For this review, take the finished solid that the model builds, in its own axes (mm). Give positions to 0.01 mm unless a question says otherwise; leave off trailing zeros. Loops run counter-clockwise (first coordinate to the right, second up) from the corner with the lowest first, then second, coordinate; pieces in that order, holes last. Notation, with made-up numbers: M -38,76.5 L 14,76.5 A6 ccw 14,86.5 Z; hole C -4.5,61.25 d3. An arc over 180 degrees is marked long. Use CSV: the item, a comma, the result in double quotes. Start each with the question number.
1. Take a section at C-C, the plane x = -6. Write out the cut boundary in (y, z), and give its area (3 significant figures).
2. Take a section at B-B, the plane y = 10. Write out the cut boundary in (x, z).
3. To check wall thickness, follow line 1 (X direction, y = 6, z = 9.5); line 2 (X direction, y = 13, z = 50); line 3 (X direction, y = 3.5, z = 80). State the ranges of each line that lie inside material, in increasing order. Write a range as [from, to].
4. Take a section at A-A, the plane z = 85. Write out the cut boundary in (x, y).
5. Take a section at D-D, the plane z = 40. Write out the cut boundary in (x, y), and give its area (3 significant figures).
6. Insertion check: P1, Ø6, axis at y = 8, z = 85, coming from the +X side. The pin has a flat end and moves straight along its axis. Give the tip position at first contact, or say it passes through.
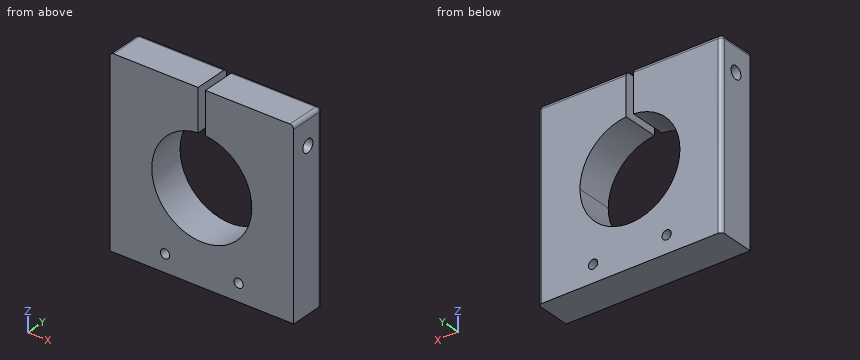
from build123d import *

# Parameters (mm, degrees)
BOSS_EXTRU_1_DEPTH      = 20
ESQUISSE2_R             = 27.2
ENL_V_MAT_EXTRU_1_DEPTH = 20
ESQUISSE3_R             = 2.5
ENL_V_MAT_EXTRU_2_DEPTH = 20
ESQUISSE4_R             = 3.5
ENL_V_MAT_EXTRU_3_DEPTH = 143.828568571
CONG_1_R                = 2


with BuildPart() as part:
    # Esquisse1 → Boss.-Extru.1 (new body)
    with BuildSketch(Plane(origin=(0, 0, 0), x_dir=(1, 0, 0), z_dir=(0, 1, 0))):
        Polygon((0, 0), (50, 0), (50, -100), (2, -100), (2, -50), (0, -50), align=None)
    boss_extru_1 = extrude(amount=BOSS_EXTRU_1_DEPTH)

    # Symétrie1: Boss.-Extru.1 across plane
    add(boss_extru_1.mirror(Plane(origin=(0, 0, 0), x_dir=(0, 0, 1), z_dir=(1, 0, 0))))

    # Esquisse2 → Enlèv. mat.-Extru.1 (cut)
    with BuildSketch(Plane(origin=(0, 20, 0), x_dir=(1, 0, 0), z_dir=(0, 1, 0))):
        with Locations((0, -50)):
            Circle(ESQUISSE2_R)
    extrude(amount=-ENL_V_MAT_EXTRU_1_DEPTH, mode=Mode.SUBTRACT)

    # Esquisse3 → Enlèv. mat.-Extru.2 (cut)
    with BuildSketch(Plane(origin=(0, 20, 0), x_dir=(1, 0, 0), z_dir=(0, 1, 0))):
        with Locations(Location((20, -9.5, 0), (0, 0, 270))):
            Circle(ESQUISSE3_R)
    enl_v_mat_extru_2 = extrude(amount=-ENL_V_MAT_EXTRU_2_DEPTH, mode=Mode.SUBTRACT)

    # Symétrie3: Enlèv. mat.-Extru.2 across plane
    add(enl_v_mat_extru_2.mirror(Plane(origin=(0, 0, 0), x_dir=(0, 0, 1), z_dir=(1, 0, 0))), mode=Mode.SUBTRACT)

    # Esquisse4 → Enlèv. mat.-Extru.3 (cut, through all)
    with BuildSketch(Plane(origin=(50, 0, 0), x_dir=(0, 0, -1), z_dir=(1, 0, 0))):
        with Locations((-85, 10)):
            Circle(ESQUISSE4_R)
    extrude(amount=-ENL_V_MAT_EXTRU_3_DEPTH, mode=Mode.SUBTRACT)

    # Congé1
    cong_1_edges = [part.edges().sort_by_distance(p)[0] for p in [
        (50, 10, 100),
        (26, 20, 100),
        (50, 20, 50),
        (-50, 20, 50),
        (-26, 20, 100),
        (-50, 10, 100),
    ]]
    fillet(cong_1_edges, radius=CONG_1_R)


solid = part.part
Result set:
1,outline,"M 0,0 L 20,0 L 20,23.47 L 0,23.47 Z; M 0,76.53 L 20,76.53 L 20,98 A2 ccw 18,100 L 0,100 Z; hole C 10,85 d7"
1,area,"899 mm2"
2,outline,"M -50,0 L 50,0 L 50,81.5 L 2,81.5 L 2,77.13 A27.2 cw long -2,77.13 L -2,81.5 L -50,81.5 Z; M -50,88.5 L -2,88.5 L -2,100 L -48,100 A2 ccw -50,98 Z; M 2,88.5 L 50,88.5 L 50,98 A2 ccw 48,100 L 2,100 Z; hole C -20,9.5 d5; hole C 20,9.5 d5"
3,line 1,"[-50, -22.5], [-17.5, 17.5], [22.5, 50]"
3,line 2,"[-50, -27.2], [27.2, 50]"
3,line 3,"[-50, -2], [2, 50]"
4,outline,"M -50,0 L -2,0 L -2,6.5 L -50,6.5 Z; M -50,13.5 L -2,13.5 L -2,20 L -48,20 A2 ccw -50,18 Z; M 2,0 L 50,0 L 50,6.5 L 2,6.5 Z; M 2,13.5 L 50,13.5 L 50,18 A2 ccw 48,20 L 2,20 Z"
5,outline,"M -50,0 L -25.3,0 L -25.3,20 L -48,20 A2 ccw -50,18 Z; M 25.3,0 L 50,0 L 50,18 A2 ccw 48,20 L 25.3,20 Z"
5,area,"986 mm2"
6,P1,"x = 50"
